```python
from build123d import *

# Parameters (mm, degrees)
SKETCH1_R           = 3.3782
BOSS_EXTRUDE1_DEPTH = 3.175
CHAMFER1_SIZE       = 3.175


with BuildPart() as part:
    # Sketch1 → Boss-Extrude1 (new body)
    with BuildSketch(Plane(origin=(0, 0, 0), x_dir=(0, 0, -1), z_dir=(1, 0, 0))):
        with BuildLine():
            Line((0, 0), (0, 38.1))
            ThreePointArc((0, 38.1), (5.363098697, 60.818450651), (20.32, 78.74))
            Line((20.32, 78.74), (81.28, 124.46))
            ThreePointArc((81.28, 124.46), (97.702892705, 123.454183744), (99.350249741, 107.083194588))
            Line((99.350249741, 107.083194588), (25.4, 0))
            Line((25.4, 0), (0, 0))
        make_face()
        with Locations((12.7, 9.525)):
            Circle(SKETCH1_R, mode=Mode.SUBTRACT)
        with Locations((12.7, 28.575)):
            Circle(SKETCH1_R, mode=Mode.SUBTRACT)
    extrude(amount=BOSS_EXTRUDE1_DEPTH)

    # Chamfer1
    chamfer1_edges = [part.edges().sort_by_distance(p)[0] for p in [
        (1.5875, 0, 0),
    ]]
    chamfer(chamfer1_edges, length=CHAMFER1_SIZE)


solid = part.part
```
Part model, mm, in its own coordinate system. Coordinates: 2 decimals unless noted, no trailing zeros. Write each loop counter-clockwise with the first axis right and the second up, starting at its lowest first coordinate (ties: lowest second). Pieces come first, ordered by that corner, then holes.
Item 1: Pin check, flat tips, straight feed: pin 1 (1 mm diameter, centred on x = 1, z = -81, fed in from +Y); pin 2 (1 mm diameter, centred on x = 2, z = -42.5, fed in from +Y). Stop position of each tip, or through.
Item 2: Slice it at C-C (y = 115). Write the cut outline in (x, z) (3 decimals), and give its area (3 significant figures).
Item 3: Mould opens along Y. For faces 1 (the face through (1.565, 60.523, -5.217)), 2 (the face through (1.565, 1.565, -1.61)), 3 (the face through (1.565, 31.924, -12.26)), 4 (the face through (2, 20, 0)) say: released by +Y, released by -Y, zero draft, split by the parting line, or undercut.
Item 4: Slice it at D-D (z = -73). Write the cut outline in (x, y) (3 decimals).
Item 5: Probe line 1 (Y direction, x = 2.4, z = -12.7); line 2 (Y direction, x = 1.8, z = -73); line 3 (Y direction, x = 0.75, z = -18). List the from-to ranges inside material, lowest first.
Item 6: Slice it at B-B (z = -12.7). Write the cut outline in (x, y) (3 decimals), and give its area (3 significant figures).
Item 7: Slice it at A-A (x = 2.5). Write the cut outline in (y, z) (3 decimals).
Results found:
1. pin 1: stops at y = 124.62
1. pin 2: stops at y = 95.75
2. outline: (0, -101.581) - (3.175, -101.581) - (3.175, -68.667) - (0, -68.667) - close
2. area: 105 mm2
3. face 1: released by +Y
3. face 2: released by -Y
3. face 3: undercut
3. face 4: zero draft
4. outline: (0, 68.927) - (3.175, 68.927) - (3.175, 118.25) - (0, 118.25) - close
5. line 1: y = 0 to 6.15, 12.9 to 25.2, 31.95 to 71.7
5. line 2: y = 68.93 to 118.25
5. line 3: y = 0 to 76.89
6. outline: (0, 0) - (3.175, 0) - (3.175, 6.147) - (0, 6.147) - close; (0, 12.903) - (3.175, 12.903) - (3.175, 25.197) - (0, 25.197) - close; (0, 31.953) - (3.175, 31.953) - (3.175, 71.701) - (0, 71.701) - close
6. area: 185 mm2
7. outline: (0, -25.4) - (107.083, -99.35) arc R12.7 ccw to (124.46, -81.28) - (78.74, -20.32) arc R50.8 ccw to (38.1, 0) - (3.175, 0) - (0, -3.175) - close; hole circle Ø6.756 at (9.525, -12.7); hole circle Ø6.756 at (28.575, -12.7)
